Source: three-view drawing plus pictorial views. Frame: mm from the lowest corner of the part. Give positions to 0.01 mm unless a question says otherwise; leave off trailing zeros. Order: outer loops, then holes, each group sorted by start corner. A loop starts at its lowest first (then second) coordinate and runs counter-clockwise, first axis right, second up. Notation, with made-up numbers: (-3.75, 56) -> (4.25, 56) arc R16 cw to (4.25, 66) -> close; hole circle Ø10 at (38, 9). An arc over 180 degrees is marked (long way). One line per question, with ' | ' between items.
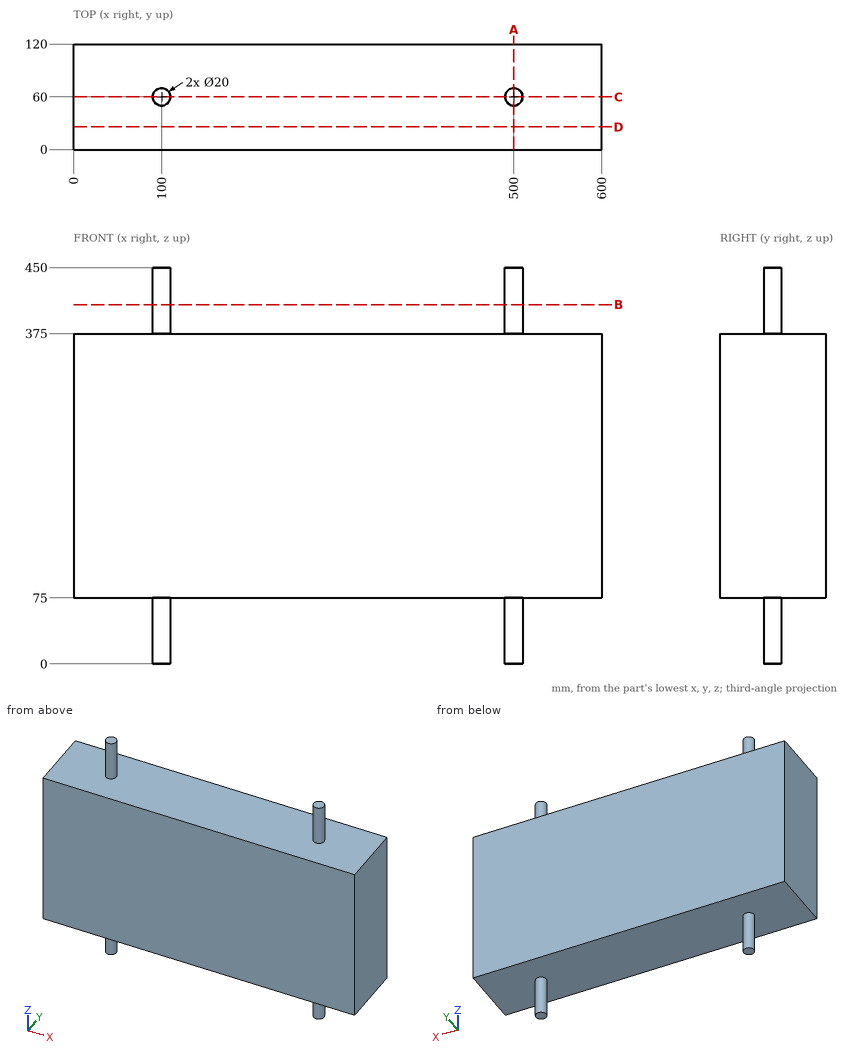
1) Section C-C on y = 60. Return loops of the section in (x, z).
Check result:
outline: (0, 75) -> (90, 75) -> (90, 0) -> (110, 0) -> (110, 75) -> (490, 75) -> (490, 0) -> (510, 0) -> (510, 75) -> (600, 75) -> (600, 375) -> (510, 375) -> (510, 450) -> (490, 450) -> (490, 375) -> (110, 375) -> (110, 450) -> (90, 450) -> (90, 375) -> (0, 375) -> close
2) Section A-A on x = 500. Return loops of the section in (y, z), plus the area to 3 significant figures.
Check result:
outline: (0, 75) -> (50, 75) -> (50, 0) -> (70, 0) -> (70, 75) -> (120, 75) -> (120, 375) -> (70, 375) -> (70, 450) -> (50, 450) -> (50, 375) -> (0, 375) -> close | area: 39,000 mm^2
3) Section D-D on y = 26. Return loops of the section in (x, z), plus the area to 3 significant figures.
Check result:
outline: (0, 75) -> (600, 75) -> (600, 375) -> (0, 375) -> close | area: 180,000 mm^2
4) Section B-B on z = 408. Return loops of the section in (x, y), plus the area to 3 significant figures.
Check result:
outline: circle Ø20 at (100, 60); circle Ø20 at (500, 60) | area: 628 mm^2
5) Material intervals for probe 1 along X at (y, z) = (61.5, 390.5); probe 2 along Z at (x, y) = (434, 28.5), sorted ascending. Write a range as from..to.
Check result:
probe 1: x = 90.11..109.89, 490.11..509.89 | probe 2: z = 75..375
6) Contact query for flat-ended pins moving along their axis: pin 1 Ø1.5 at (x, y) = (305.5, 31.5) entering from +Z; pin 2 Ø1 at (x, y) = (193.5, 88) entering from -Z. Output: stop coordinate, or through.
Check result:
pin 1: stops at z = 375 | pin 2: stops at z = 75
